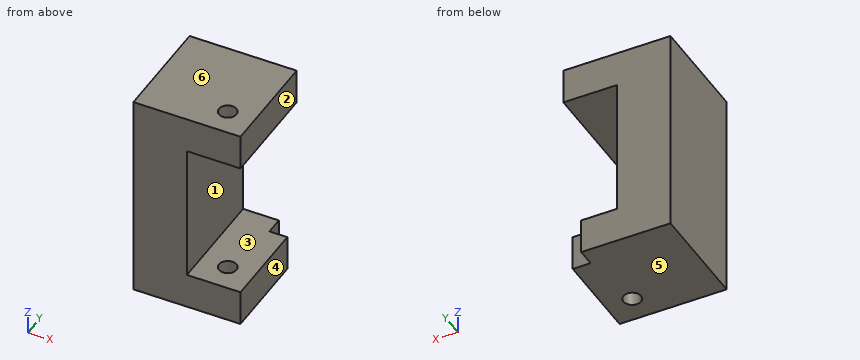
Autodesk Inventor part; units mm, degrees
ref_plane "YZ Plane" through (0, 0, 0) normal (1, 0, 0) x (0, 1, 0)
ref_plane "XZ Plane" through (0, 0, 0) normal (0, 1, 0) x (-1, 0, 0)
ref_plane "XY Plane" through (0, 0, 0) normal (0, 0, 1) x (1, 0, 0)
sketch "Skizze1" plane through (0, 0, 0) normal (0, 1, 0) x (-1, 0, 0)
  line L0 (3.7731, -4.4076) -> (3.7731, -12.4076)
  line L1 (10.7449, 21.0924) -> (18.7731, 21.0924)
  line L2 (18.7731, 21.0924) -> (18.7731, -37.9076)
  line L3 (18.7731, -37.9076) -> (10.7449, -37.9076)
  line L4 (10.7449, 21.0924) -> (-11.2269, 21.0924)
  line L5 (-11.2269, 21.0924) -> (-11.2269, 11.0924)
  line L6 (-11.2269, 11.0924) -> (3.7731, 11.0924)
  line L7 (10.7449, -37.9076) -> (-11.2269, -37.9076)
  line L8 (-11.2269, -37.9076) -> (-11.2269, -27.9076)
  line L9 (-11.2269, -27.9076) -> (3.7731, -27.9076)
  line L10 (3.7731, -12.4076) -> (3.7731, -12.4076)
  line L11 (3.7731, -4.4076) -> (3.7731, -4.4076)
  line L12 (3.7731, -27.9076) -> (3.7731, -12.4076)
  line L13 (3.7731, -4.4076) -> (3.7731, 11.0924)
  point P0 (0, 0)
  dimension "d1" = 15
  dimension "d2" = 15.5
  dimension "d3" = 15.5
  dimension "d5" = 10
  dimension "d6" = 59
  dimension "d7" = 0
  dimension "d8" = 15
  dimension "d64" = 8
  dimension "d65" = 10
extrude "Extrusion1" add sketch "Skizze1" along normal blind 30
sketch "Skizze2" plane through (0, 30, 0) normal (0, 1, 0) x (1, 0, 0)
  line L0 (11.2269, 27.9076) -> (11.2269, 37.9076)
  line L1 (11.2269, 37.9076) -> (6.2269, 37.9076)
  line L2 (6.2269, 37.9076) -> (6.2269, 27.9076)
  line L3 (6.2269, 27.9076) -> (11.2269, 27.9076)
  line L4 (11.2269, 27.9076) -> (11.2269, 37.9076)
  line L5 (-3.7731, 27.9076) -> (11.2269, 27.9076)
  point P0 (0, 0)
  dimension "d11" = 0
  dimension "d12" = 5
extrude "Extrusion2" cut sketch "Skizze2" against normal blind 5
sketch "Skizze6" plane through (-18.7731, 0, 21.0924) normal (0, 0, 1) x (1, 0, 0)
  circle A0 centre (22.5, 7.5) radius 4.6596
  line L0 (30, 0) -> (0, 0)
  line L1 (30, 0) -> (30, 30)
  point P0 (18.7731, 0)
  dimension "d27" = 7.5
  dimension "d28" = 7.5
hole "Bohrung1" at (3.7269, 7.5, 21.0924) direction (0, 0, -1) diameter 4.917 depth 17 tip angle 118
sketch "Skizze8" plane through (11.2269, 0, -37.9076) normal (0, 0, -1) x (-1, 0, 0)
  circle A0 centre (7.5, 7.5) radius 1.9257
  line L0 (30, 0) -> (0, 0)
  line L1 (0, 0) -> (0, 25)
  point P0 (11.2269, 0)
  dimension "d45" = 7.5
  dimension "d46" = 7.5
hole "Bohrung3" at (3.7269, 7.5, -37.9076) direction (0, 0, 1) diameter 4.917 depth 17 tip angle 118
properties material "Nylon 6"
Geometry: final body of the model. Coordinates: model frame, mm. Face numbers are marked on the shaded views. A direction names the side the tool comes from. Give positions to 0.01 mm unless a question says otherwise; leave off trailing zeros. Order: outer loops, then holes, each group sorted by start corner. A loop starts at its lowest first (then second) coordinate and runs counter-clockwise, first axis right, second up. Notation, with made-up numbers: (-24, 1.25) -> (0, 1.25) arc R30 ccw to (0, 31.25) -> close; hole circle Ø2 at (-7.75, -15.5). An arc over 180 degrees is marked (long way). Write each question's results on one line, items separated by ' | '.
1) Cut plane C-C (y = 17). Output: boundary loops of the cut face in (x, z), and give its area (4 significant figures).
Geometry says:
outline: (-18.77, -37.91) -> (11.23, -37.91) -> (11.23, -27.91) -> (-3.77, -27.91) -> (-3.77, 11.09) -> (11.23, 11.09) -> (11.23, 21.09) -> (-18.77, 21.09) -> close | area: 1,185 mm²
2) Cut plane B-B (y = 7.5). Output: boundary loops of the cut face in (x, z), and give its area (3 significant figures).
Geometry says:
outline: (-18.77, -37.91) -> (1.27, -37.91) -> (1.27, -27.91) -> (-3.77, -27.91) -> (-3.77, 11.09) -> (1.27, 11.09) -> (1.27, 21.09) -> (-18.77, 21.09) -> close; (6.19, -37.91) -> (11.23, -37.91) -> (11.23, -27.91) -> (6.19, -27.91) -> close; (6.19, 11.09) -> (11.23, 11.09) -> (11.23, 21.09) -> (6.19, 21.09) -> close | area: 1,090 mm²
3) Line query: line 1 along Z through (x, y) = (5.25, 9.5); line 2 along X through (y, z) = (7.5, -34.75); line 3 along X through (y, z) = (2, 2). Output: solid intervals per line, ascending.
Geometry says:
line 1: z = -37.91 to -27.91, 11.09 to 21.09 | line 2: x = -18.77 to 1.27, 6.19 to 11.23 | line 3: x = -18.77 to -3.77
4) Cut plane A-A (x = 8.5). Output: boundary loops of the cut face in (y, z), and give its area (3 significant figures).
Geometry says:
outline: (0, -37.91) -> (25, -37.91) -> (25, -27.91) -> (0, -27.91) -> close; (0, 11.09) -> (30, 11.09) -> (30, 21.09) -> (0, 21.09) -> close | area: 550 mm²
5) First-contact query: pin 1 Ø3 at (x, y) = (3.73, 7.5) entering from +Z; pin 2 Ø2.5 at (y, z) = (28.5, -35) entering from +X; pin 3 Ø8 at (y, z) = (9, -18.5) entering from +X; pin 4 Ø2 at (x, z) = (8, -27.5) entering from +Y. Flat tips, straight axial feed; report the tip coordinate or a pass-through.
Geometry says:
pin 1: passes through | pin 2: stops at x = 6.23 | pin 3: stops at x = -3.77 | pin 4: stops at y = 25
6) Cut plane D-D (z = 14.5). Output: boundary loops of the cut face in (x, y), and give its area (3 significant figures).
Geometry says:
outline: (-18.77, 0) -> (11.23, 0) -> (11.23, 30) -> (-18.77, 30) -> close; hole circle Ø4.92 at (3.73, 7.5) | area: 881 mm²
7) Draft query along Z for the marked faces 3, 4, 5 and 6. Return one class per face: released by +Z, released by -Z, zero draft, split by the parting line, or undercut.
Geometry says:
face 3: undercut | face 4: zero draft | face 5: released by -Z | face 6: released by +Z
8) Set-up query: the marked faces 1 and 2. Return all of +Z, -Z, +X, -X, +Y, -Y with unobstructed straight access to the full face (end or side cutting, diameter ignored); none if empty.
Geometry says:
face 1: +X, +Y, -Y | face 2: +Z, -Z, +X, +Y, -Y
